For this review, take the finished solid that the model builds, in its own axes (mm). Face numbers are marked on the shaded views. A direction names the side the tool comes from. Give positions to 0.01 mm unless a question says otherwise; leave off trailing zeros. Write each loop counter-clockwise with the first axis right and the second up, starting at its lowest first coordinate (ties: lowest second). Pieces come first, ordered by that corner, then holes. Notation, with made-up numbers: (-28, 7) -> (-11, 7) arc R17 ccw to (-11, 18) -> close; hole circle Ø4 at (23.25, 84.25). An arc over 180 degrees is marked (long way). Write item = value, one per line.
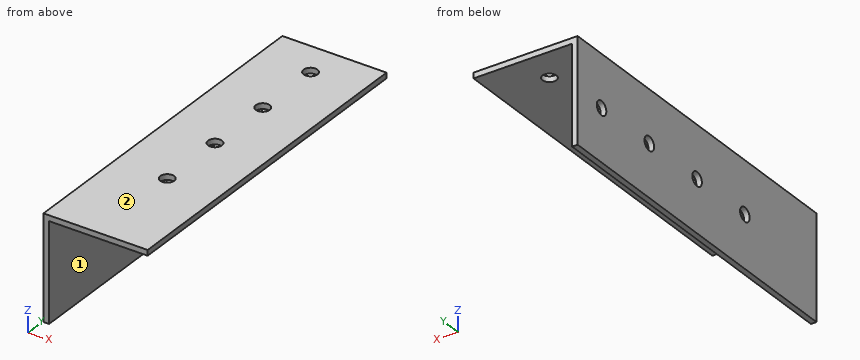
```python
from build123d import *

# Parameters (mm, degrees)
EXTRUDE_1_DEPTH     = 250
SKETCH_2_R          = 5
CUT_EXTRUDE_1_DEPTH = 10
SKETCH_3_R          = 5
CUT_EXTRUDE_2_DEPTH = 10


with BuildPart() as part:
    # Эскиз1 → Вытянуть-Тонкостенный1 (new body)
    with BuildSketch(Plane(origin=(0, 0, 0), x_dir=(1, 0, 0), z_dir=(0, 1, 0))):
        Polygon((0, 75), (0, 0), (75, 0), (75, 4), (4, 4), (4, 75), align=None)
    extrude(amount=EXTRUDE_1_DEPTH)

    # Эскиз2 → Вырез-Вытянуть1 (cut)
    with BuildSketch(Plane.XY):
        with Locations((37.5, 225)):
            Circle(SKETCH_2_R)
        with Locations((37.5, 175)):
            Circle(SKETCH_2_R)
        with Locations((37.5, 125)):
            Circle(SKETCH_2_R)
        with Locations((37.5, 75)):
            Circle(SKETCH_2_R)
    extrude(amount=-CUT_EXTRUDE_1_DEPTH, mode=Mode.SUBTRACT)

    # Эскиз3 → Вырез-Вытянуть2 (cut)
    with BuildSketch(Plane.ZY):
        with Locations((-37.5, 225)):
            Circle(SKETCH_3_R)
        with Locations((-37.5, 175)):
            Circle(SKETCH_3_R)
        with Locations((-37.5, 125)):
            Circle(SKETCH_3_R)
        with Locations((-37.5, 75)):
            Circle(SKETCH_3_R)
    extrude(amount=-CUT_EXTRUDE_2_DEPTH, mode=Mode.SUBTRACT)


solid = part.part
```
(1) Take a section at D-D (x = 14). Write out the cut boundary in (y, z), plus the area to 3 significant figures.
Answers below:
outline = (0, -4) -> (250, -4) -> (250, 0) -> (0, 0) -> close
area = 1,000 mm^2
(2) To check wall thickness, follow probe 1 along Y at (x, z) = (37.5, -2); probe 2 along Z at (x, y) = (7.5, 29.5); probe 3 along X at (y, z) = (83.5, -22). State the ranges of each line that lie inside material, in increasing order.
Answers below:
probe_1 = 0 to 70, 80 to 120, 130 to 170, 180 to 220, 230 to 250
probe_2 = -4 to 0
probe_3 = 0 to 4
(3) Take a section at B-B (z = -37.5). Write out the cut boundary in (x, y).
Answers below:
outline = (0, 0) -> (4, 0) -> (4, 70) -> (0, 70) -> close; (0, 80) -> (4, 80) -> (4, 120) -> (0, 120) -> close; (0, 130) -> (4, 130) -> (4, 170) -> (0, 170) -> close; (0, 180) -> (4, 180) -> (4, 220) -> (0, 220) -> close; (0, 230) -> (4, 230) -> (4, 250) -> (0, 250) -> close
(4) Take a section at A-A (y = 225). Write out the cut boundary in (x, z), plus the area to 3 significant figures.
Answers below:
outline = (0, -75) -> (4, -75) -> (4, -42.5) -> (0, -42.5) -> close; (0, -32.5) -> (4, -32.5) -> (4, -4) -> (32.5, -4) -> (32.5, 0) -> (0, 0) -> close; (42.5, -4) -> (75, -4) -> (75, 0) -> (42.5, 0) -> close
area = 504 mm^2
(5) Take a section at C-C (y = 23.5). Write out the cut boundary in (x, z).
Answers below:
outline = (0, -75) -> (4, -75) -> (4, -4) -> (75, -4) -> (75, 0) -> (0, 0) -> close
(6) For pin 1 (13 mm diameter, centred on y = 125, z = -37.5, fed in from +X); pin 2 (21.5 mm diameter, centred on x = 49, y = 176, fed in from -Z); pin 3 (1.5 mm diameter, centred on y = 175, z = -50.5, fed in from -X), all flat-tipped, find the tip position at first contact; note any pin that passes through.
Answers below:
pin_1 = 4
pin_2 = -4
pin_3 = 0
(7) Tool access review of the marked faces 1 and 2: name each direction out of +Z, -Z, +X, -X, +Y, -Y from which nothing blocks a thin tool from reaching the whole face with its end or side.
Answers below:
face_1 = -Z, +X, +Y, -Y
face_2 = +Z, +X, -X, +Y, -Y
